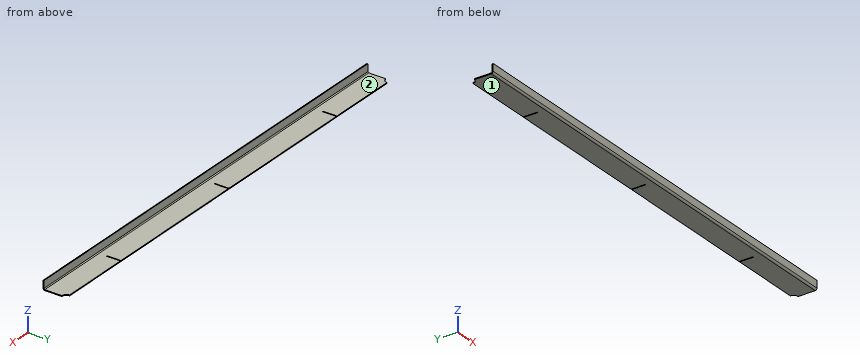
Autodesk Inventor part; units mm, degrees
ref_plane "YZ Plane" through (0, 0, 0) normal (1, 0, 0) x (0, 1, 0)
ref_plane "XZ Plane" through (0, 0, 0) normal (0, 1, 0) x (-1, 0, 0)
ref_plane "XY Plane" through (0, 0, 0) normal (0, 0, 1) x (1, 0, 0)
sketch "Sketch1" plane through (0, 0, 0) normal (0, 0, 1) x (1, 0, 0)
  line L0 (-750, 77.5094) -> (750, 77.5094)
  line L1 (750, 77.5094) -> (750, 0)
  line L2 (750, 0) -> (-750, 0)
  line L3 (-750, 0) -> (-750, 77.5094)
  point P0 (0, 0)
  point P1 (0, 0)
  dimension "d0" = 1500
  dimension "d1" = 77.5094
extrude "Plate1" add sketch "Sketch1" along normal blind 3
sketch "Sketch2" plane through (750, 3, 0) normal (0, -1, 0) x (1, 0, 0)
  line L0 (-1500, 0) -> (0, 0)
  line L1 (0, 0) -> (0, 30)
  line L2 (0, 30) -> (-1500, 30)
  line L3 (-1500, 30) -> (-1500, 0)
edge flange "Flange1" height 30 angle 90 thickness 3 bend radius 3 thickness toward (0, -1, 0) relief tear relief width 3 relief depth 1.5 edges at (0, 0, 3) wall of the first edge with corners at (-750, 3, 0) (750, 3, 0) (750, 3, 30) (-750, 3, 30)
bend "Bend1"
corner "Corner1"
sketch "Sketch5" plane through (0, 0, 0) normal (0, 0, -1) x (-1, 0, 0)
  line L0 (750, 77.5094) -> (-750, 77.5094)
  line L1 (500, 77.5094) -> (500, 31)
  line L2 (500, 31) -> (503, 31)
  line L3 (503, 31) -> (503, 77.5094)
  line L4 (750, 0) -> (-750, 0)
  point P0 (0, 0)
  dimension "d18" = 3
  dimension "d19" = 247
  dimension "d20" = 31
extrude "Extrusion1" cut sketch "Sketch5" against normal through all
pattern_linear "Rectangular Pattern1" count 3 spacing 500 along (1, 0, 0) of "Extrusion1"
sketch "Sketch6" plane through (0, 0, 0) normal (0, 0, -1) x (-1, 0, 0)
  line L0 (-750, 77.5094) -> (-750, 6)
  circle A0 centre (-750, 77.5094) radius 15
  line L1 (-750, 77.5094) -> (-500, 77.5094)
  point P0 (0, 0)
  point P1 (-735, 77.5094)
  point P2 (-750, 62.5094)
  dimension "d24" = 30
extrude "Extrusion2" cut sketch "Sketch6" against normal through all contours L1 A0 L0 picked at (-740.1254, 76.3968)
mirror "Mirror1" about plane through (0, 0, 0) normal (1, 0, 0) of "Extrusion2"
equation "\"d1\" = Стрингер_6"
equation "\"d18\" = Thickness"
equation "\"d2\" = Thickness"
equation "\"d3\" = BendReliefWidth"
equation "\"d4\" = BendReliefDepth"
equation "\"d5\" = MinimumRemnant"
equation "\"d6\" = TransitionRadius"
equation "\"d9\" = BendRadius"
equation "\"d10\" = CornerReliefSize"
equation "\"d11\" = GapSize"
equation "\"d12\" = JacobiRadiusSize"
equation "\"BendRadius\" = Thickness"
equation "\"BendReliefWidth\" = Thickness"
equation "\"BendReliefDepth\" = 0.5 * Thickness"
equation "\"CornerReliefSize\" = 4 * Thickness"
equation "\"MinimumRemnant\" = 2 * Thickness"
equation "\"TransitionRadius\" = BendRadius"
equation "\"JacobiRadiusSize\" = BendRadius"
equation "\"GapSize\" = Thickness"
properties part number "МОО 056 стрингер борт 61"
Geometry check sheet. Reference: the model listing, model coordinates, mm. Face numbers are marked on the shaded views. A direction names the side the tool comes from. Give positions to 0.01 mm unless a question says otherwise; leave off trailing zeros. Order: outer loops, then holes, each group sorted by start corner. A loop starts at its lowest first (then second) coordinate and runs counter-clockwise, first axis right, second up.
1) Cross-section at B-B (z = 14). Record the boundary of the cut face in (x, y), then the cut area to 3 significant figures.
Results are:
outline: (-750, 0) - (750, 0) - (750, 3) - (-750, 3) - close
area: 4,500 mm2
2) Gauge pin test, flat ends, axial feed: pin 1 (0.9 mm diameter, centred on x = 499, z = 1, fed in from +Y); pin 2 (1.5 mm diameter, centred on x = 335.5, y = 36.5, fed in from +Z); pin 3 (8 mm diameter, centred on x = -597, z = 23, fed in from -Y). Record the tip position at first contact, or that the pin passes through.
Results are:
pin 1: stops at y = 31
pin 2: stops at z = 3
pin 3: stops at y = 0
3) Cross-section at A-A (x = 650). Record the boundary of the cut face in (y, z), then the cut area to 3 significant figures.
Results are:
outline: (0, 6) arc R6 ccw to (6, 0) - (77.51, 0) - (77.51, 3) - (6, 3) arc R3 cw to (3, 6) - (3, 30) - (0, 30) - close
area: 308 mm2
4) Material ranges on probe 1 along X at (y, z) = (34, 2.25); probe 2 along Z at (x, y) = (569, 59), recorded low to high.
Results are:
probe 1: x = -750 to -503, -500 to -3, 0 to 497, 500 to 750
probe 2: z = 0 to 3
5) Tool access check on the marked faces 1 and 2. Record the directions out of +Z, -Z, +X, -X, +Y, -Y that give a thin tool (end or side, any length) a straight path to the whole face; none if there is none.
Results are:
face 1: -Z, +X, -X, +Y, -Y
face 2: +Z, +X, -X, +Y
